Part model, mm, in its own coordinate system. Round coordinates to 2 decimals unless told otherwise and drop trailing zeros. Write each loop counter-clockwise with the first axis right and the second up, starting at its lowest first coordinate (ties: lowest second). Pieces come first, ordered by that corner, then holes. Notation, with made-up numbers: M 19,-20.75 L 50,-20.75 A22 cw 50,-14.75 Z; hole C -38.75,86 d7. An arc over 180 degrees is marked long. Use one line per item in the form item = value. Start each with the question number.
Item 1: Cut at C-C, the plane x = 17.75. Give the cut face in (y, z), then the cut area to 3 significant figures.
Item 2: Flat gauge pins, fed straight in: pin 1 Ø1 at (x, z) = (5.5, 11) entering from +Y; pin 2 Ø4 at (x, z) = (5.5, -14) entering from -Y; pin 3 Ø6 at (x, z) = (15.5, 15) entering from +Y. Where does each tip first touch, or does it go through?
Item 3: Cut at D-D, the plane x = 4.75. Give the cut face in (y, z), then the cut area to 3 significant figures.
Item 4: Mould opens along Z. For faces 1 (the face through (0, -13, 0)), 2 (the face through (10.14, 3.755, -11.923)) say: +Z half, -Z half, draft (parallel to the pull), parting line (faces both ways), or undercut.
Item 5: Probe L1, parallel to Y at x = 10.5, z = 0; L2, parallel to Y at x = 14, z = 0; L3, parallel to Z at x = 15.5, y = -3. List the from-to ranges inside material, lowest first.
from build123d import *

# Parameters (mm, degrees)
SKETCH1_R           = 40
BOSS_EXTRUDE1_DEPTH = 20
FILLET2_R           = 10
SKETCH2_R           = 12.5
CUT_EXTRUDE1_DEPTH  = 20


with BuildPart() as part:
    # Sketch1 → Boss-Extrude1 (new body)
    with BuildSketch(Plane(origin=(0, 0, 0), x_dir=(0, 0, -1), z_dir=(1, 0, 0))):
        Circle(SKETCH1_R)
    extrude(amount=BOSS_EXTRUDE1_DEPTH)

    # Fillet2
    fillet2_edges = [part.edges().sort_by_distance(p)[0] for p in [
        (0, 0, 40),
        (20, 0, 40),
    ]]
    fillet(fillet2_edges, radius=FILLET2_R - 0.0001)  # a hair under: the kernel refuses the full size

    # Sketch2 → Cut-Extrude1 (cut)
    with BuildSketch(Plane(origin=(20, 0, 0), x_dir=(0, 0, -1), z_dir=(1, 0, 0))):
        Circle(SKETCH2_R)
    extrude(amount=-CUT_EXTRUDE1_DEPTH, mode=Mode.SUBTRACT)


solid = part.part
Model answer:
q1.outline = C 0,0 d72.64; hole C 0,0 d25
q1.area = 3,650 mm²
q2.pin_1 = 37.63
q2.pin_2 = -37.45
q2.pin_3 = 37.25
q3.outline = C 0,0 d77.02; hole C 0,0 d25
q3.area = 4,170 mm²
q4.face_1 = draft
q4.face_2 = undercut
q5.L1 = -39.99 to -12.5, 12.5 to 39.99
q5.L2 = -39.17 to -12.5, 12.5 to 39.17
q5.L3 = -38.23 to -12.13, 12.13 to 38.23
